Here's how the part is built. I have some questions about the finished solid (model axes, mm). Face numbers are marked on the shaded views. A direction names the side the tool comes from. Give positions to 0.01 mm unless a question says otherwise; leave off trailing zeros. Loops run counter-clockwise (first coordinate to the right, second up) from the corner with the lowest first, then second, coordinate; pieces in that order, holes last. Notation, with made-up numbers: (5.5, 52.25) - (34.5, 52.25) arc R29 cw to (34.5, 75.25) - close; hole circle Ø2 at (5, 42.5). An arc over 180 degrees is marked (long way). Use one line per item in the form item = value.
from build123d import *

# Parameters (mm, degrees)
SKETCH2_W             = 39.3827
SKETCH2_H             = 7.62
BOSS_EXTRUDE2_DEPTH   = 4.064
BOSS_EXTRUDE2_2_DEPTH = 4.064
BOSS_EXTRUDE3_DEPTH   = 2.54
BOSS_EXTRUDE4_DEPTH   = 38.1
SKETCH4_W             = 10.16
SKETCH4_H             = 3.81
CUT_EXTRUDE2_DEPTH    = 12.7
CUT_EXTRUDE3_REACH    = 76.205
SKETCH5_R             = 2.54
SKETCH5_R_2           = 1.143
CUT_EXTRUDE5_DEPTH    = 35.56


with BuildPart() as part:
    # Sketch2 → Boss-Extrude2 (new body)
    with BuildSketch(Plane(origin=(0, 0, 0), x_dir=(1, 0, 0), z_dir=(0, 1, 0))):
        with Locations((19.69135, 3.81)):
            Rectangle(SKETCH2_W, SKETCH2_H)
    extrude(amount=BOSS_EXTRUDE2_DEPTH)



with BuildPart() as body_2:
    # Sketch2 → Boss-Extrude2 2 (new body)
    with BuildSketch(Plane(origin=(0, 0, 0), x_dir=(1, 0, 0), z_dir=(0, 1, 0))):
        with Locations((19.69135, 72.39)):
            Rectangle(SKETCH2_W, SKETCH2_H)
    extrude(amount=BOSS_EXTRUDE2_2_DEPTH)


with BuildPart() as part_1:
    add(part.part)

    add(body_2.part)  # Boss-Extrude3 merges body 2
    # Sketch2<3> → Boss-Extrude3 (add)
    with BuildSketch(Plane(origin=(0, 0, 0), x_dir=(1, 0, 0), z_dir=(0, 1, 0))):
        with BuildLine():
            Line((0, 34.29), (0, 7.62))
            Line((0, 7.62), (39.3827, 7.62))
            Line((39.3827, 7.62), (39.3827, 68.58))
            Line((39.3827, 68.58), (0, 68.58))
            Line((0, 68.58), (0, 41.91))
            ThreePointArc((0, 41.91), (3.81, 38.1), (0, 34.29))
        make_face()
    extrude(amount=BOSS_EXTRUDE3_DEPTH)

    # Sketch2<8> → Boss-Extrude4 (add)
    with BuildSketch(Plane(origin=(0, 0, 0), x_dir=(1, 0, 0), z_dir=(0, 1, 0))):
        Polygon((6.107856951, 50.038), (6.107856951, 38.1), (6.107856951, 26.162), (21.347856951, 26.162), (21.347856951, 50.038), align=None)
        Polygon((8.533414456, 31.75), (8.533414456, 38.1), (8.533414456, 44.45), (18.693414456, 44.45), (18.693414456, 31.75), align=None, mode=Mode.SUBTRACT)
    extrude(amount=BOSS_EXTRUDE4_DEPTH)

    # Sketch4 → Cut-Extrude2 (cut)
    with BuildSketch(Plane(origin=(0, 2.54, 0), x_dir=(1, 0, 0), z_dir=(0, 1, 0))):
        with Locations((13.613414456, 46.355)):
            Rectangle(SKETCH4_W, SKETCH4_H)
        with Locations((13.613414456, 29.845)):
            Rectangle(SKETCH4_W, SKETCH4_H)
    extrude(amount=CUT_EXTRUDE2_DEPTH, mode=Mode.SUBTRACT)

    # Cut-Extrude3: up to this face of the body (flat: up to its plane)
    cut_extrude3_end = Plane(part_1.part.faces().sort_by_distance((13.727856951, 20.32, -26.162))[0])
    # Sketch5 → Cut-Extrude3 (cut, up to the picked face)
    with BuildSketch(Plane(origin=(0, 0, -50.038), x_dir=(-1, 0, 0), z_dir=(0, 0, -1)), mode=Mode.PRIVATE) as cut_extrude3_sk1:
        with Locations((-13.727856951, 30.48)):
            Circle(SKETCH5_R)
    cut_extrude3_tool1 = split(extrude(cut_extrude3_sk1.sketch, amount=-CUT_EXTRUDE3_REACH, mode=Mode.PRIVATE), bisect_by=cut_extrude3_end, keep=Keep.BOTH, mode=Mode.PRIVATE)
    # Sketch5 → Cut-Extrude3 (cut, up to the picked face)
    with BuildSketch(Plane(origin=(0, 0, -50.038), x_dir=(-1, 0, 0), z_dir=(0, 0, -1)), mode=Mode.PRIVATE) as cut_extrude3_sk2:
        with Locations((-13.727856951, 19.939)):
            Circle(SKETCH5_R_2)
    cut_extrude3_tool2 = split(extrude(cut_extrude3_sk2.sketch, amount=-CUT_EXTRUDE3_REACH, mode=Mode.PRIVATE), bisect_by=cut_extrude3_end, keep=Keep.BOTH, mode=Mode.PRIVATE)
    add(cut_extrude3_tool1.solids().sort_by(Axis((13.727857, 30.48, -50.038), (0, 0, 1)))[0], mode=Mode.SUBTRACT)
    add(cut_extrude3_tool2.solids().sort_by(Axis((13.727857, 19.939, -50.038), (0, 0, 1)))[0], mode=Mode.SUBTRACT)

    # Sketch6 → Cut-Extrude5 (cut)
    with BuildSketch(Plane(origin=(0, 38.1, 0), x_dir=(1, 0, 0), z_dir=(0, 1, 0))):
        with BuildLine():
            ThreePointArc((6.107856951, 47.286333333), (6.913801458, 49.232055493), (8.859523617, 50.038))
            Line((8.859523617, 50.038), (6.107856951, 50.038))
            Line((6.107856951, 50.038), (6.107856951, 47.286333333))
        make_face()
        with BuildLine():
            ThreePointArc((18.596190284, 50.038), (20.541912444, 49.232055493), (21.347856951, 47.286333333))
            Line((21.347856951, 47.286333333), (21.347856951, 50.038))
            Line((21.347856951, 50.038), (18.596190284, 50.038))
        make_face()
        with BuildLine():
            Line((6.107856951, 26.162), (8.859523617, 26.162))
            ThreePointArc((8.859523617, 26.162), (6.913801458, 26.967944507), (6.107856951, 28.913666667))
            Line((6.107856951, 28.913666667), (6.107856951, 26.162))
        make_face()
        with BuildLine():
            Line((21.347856951, 26.162), (21.347856951, 28.913666667))
            ThreePointArc((21.347856951, 28.913666667), (20.541912444, 26.967944507), (18.596190284, 26.162))
            Line((18.596190284, 26.162), (21.347856951, 26.162))
        make_face()
    extrude(amount=-CUT_EXTRUDE5_DEPTH, mode=Mode.SUBTRACT)


solid = part_1.part
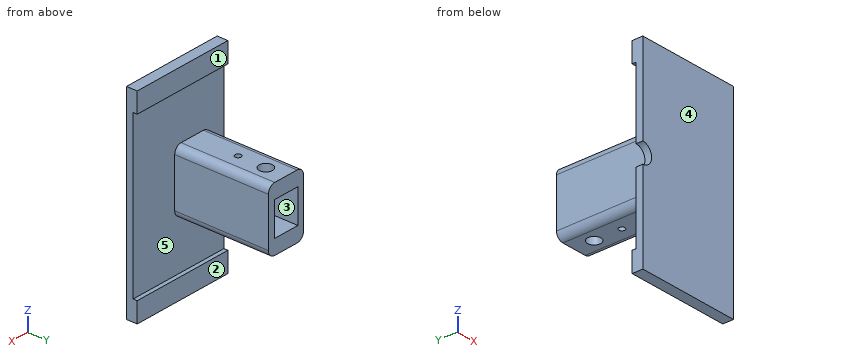
(1) If I drill on probe 1 along Z at (x, y) = (18.5, 17); probe 2 along X at (y, z) = (6, -42); probe 3 along X at (y, z) = (20, -46), over which ranges is the centre line in solid material (lowest first)?
Geometry says:
probe_1 = -50.04 to -44.45, -31.75 to -26.16
probe_2 = 6.11 to 8.53, 18.69 to 21.35
probe_3 = 6.11 to 12.59, 14.87 to 21.35
(2) If we section it at C-C (z = -43): List the corners of the cut face in (x, y) for me.
Geometry says:
outline = (0, 0) - (39.38, 0) - (39.38, 2.54) - (21.35, 2.54) - (21.35, 38.1) - (18.69, 38.1) - (18.69, 2.54) - (8.53, 2.54) - (8.53, 38.1) - (6.11, 38.1) - (6.11, 2.54) - (0, 2.54) - close
(3) If we section it at B-B (y = 35.5): List the corners of the cut face in (x, z) for me, plus the area to 3 significant figures.
Geometry says:
outline = (6.11, -47.29) arc R2.75 ccw to (8.86, -50.04) - (18.6, -50.04) arc R2.75 ccw to (21.35, -47.29) - (21.35, -28.91) arc R2.75 ccw to (18.6, -26.16) - (8.86, -26.16) arc R2.75 ccw to (6.11, -28.91) - close; hole (8.53, -44.45) - (18.69, -44.45) - (18.69, -31.75) - (8.53, -31.75) - close
area = 228 mm²
(4) Thinking about a two-plate mould opening in Z: for the marked faces 3, 4 and 5, which applies, pulls with the +Z half, pulls with the -Z half, needs draft (parallel to the pull), parting line crosses it, or undercut?
Geometry says:
face_3 = undercut
face_4 = needs draft
face_5 = undercut
(5) If we section it at D-D (x = 36): List the corners of the cut face in (y, z) for me, plus the area to 3 significant figures.
Geometry says:
outline = (0, -76.2) - (4.06, -76.2) - (4.06, -68.58) - (2.54, -68.58) - (2.54, -7.62) - (4.06, -7.62) - (4.06, 0) - (0, 0) - close
area = 217 mm²
(6) If we section it at A-A (y = 30.48): List the corners of the cut face in (x, z) for me, plus the area to 3 significant figures.
Geometry says:
outline = (6.11, -47.29) arc R2.75 ccw to (8.86, -50.04) - (11.19, -50.04) - (11.19, -44.45) - (8.53, -44.45) - (8.53, -31.75) - (11.19, -31.75) - (11.19, -26.16) - (8.86, -26.16) arc R2.75 ccw to (6.11, -28.91) - close; (16.27, -50.04) - (18.6, -50.04) arc R2.75 ccw to (21.35, -47.29) - (21.35, -28.91) arc R2.75 ccw to (18.6, -26.16) - (16.27, -26.16) - (16.27, -31.75) - (18.69, -31.75) - (18.69, -44.45) - (16.27, -44.45) - close
area = 172 mm²
(7) For the marked faces 1 and 2, which set-ups out of +Z, -Z, +X, -X, +Y, -Y let a thin tool reach every point of the face, with its end or its side?
Geometry says:
face_1 = +Z, +X, -X, +Y
face_2 = -Z, +X, -X, +Y
(8) For P1, Ø8, axis at x = 13, y = 31, coming from the -Z side; P2, Ø10.5, axis at x = 16, y = 22, coming from the +Z side; P3, Ø5.5, axis at y = 14, z = -42, coming from the -X side, each with a flat end and sliding along its axis, tell me the tip position at first contact or that it passes through.
Geometry says:
P1 = -50.04
P2 = -26.16
P3 = 6.11
